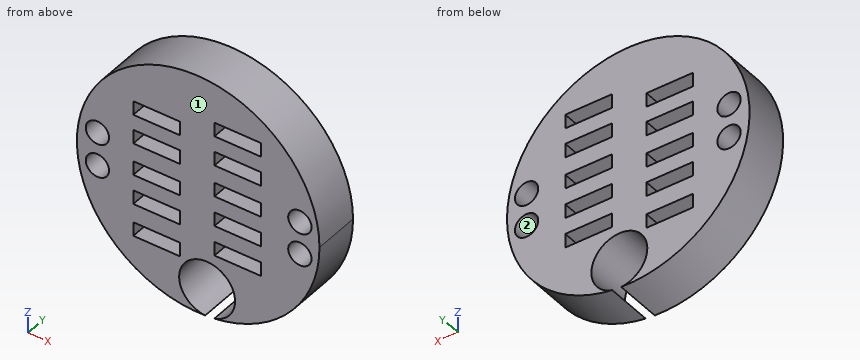
Autodesk Inventor part; units mm, degrees
ref_plane "YZ Plane" through (0, 0, 0) normal (1, 0, 0) x (0, 1, 0)
ref_plane "XZ Plane" through (0, 0, 0) normal (0, 1, 0) x (-1, 0, 0)
ref_plane "XY Plane" through (0, 0, 0) normal (0, 0, 1) x (1, 0, 0)
sketch "Sketch3" plane through (0, 0, 0) normal (0, 1, 0) x (-1, 0, 0)
  circle A0 centre (0, 0) radius 13.5
  line L0 (-6.7499, 8.6501) -> (-1.7499, 8.6501)
  line L1 (-1.7499, 8.6501) -> (-1.7499, 7.1501)
  line L2 (-1.7499, 7.1501) -> (-6.7499, 7.1501)
  line L3 (-6.7499, 7.1501) -> (-6.7499, 8.6501)
  line L4 (-6.75, 5.45) -> (-1.7499, 5.45)
  line L5 (-1.7499, 5.45) -> (-1.7499, 3.95)
  line L6 (-1.7499, 3.95) -> (-6.75, 3.95)
  line L7 (-6.75, 3.95) -> (-6.75, 5.45)
  line L8 (-6.75, 2.0498) -> (-1.75, 2.0498)
  line L9 (-1.75, 2.0498) -> (-1.75, 0.5498)
  line L10 (-1.75, 0.5498) -> (-6.75, 0.5498)
  line L11 (-6.75, 0.5498) -> (-6.75, 2.0498)
  line L12 (-6.75, -1.2) -> (-1.75, -1.2)
  line L13 (-1.75, -1.2) -> (-1.75, -2.7)
  line L14 (-1.75, -2.7) -> (-6.75, -2.7)
  line L15 (-6.75, -2.7) -> (-6.75, -1.2)
  line L16 (-6.75, -4.4501) -> (-1.75, -4.4501)
  line L17 (-1.75, -4.4501) -> (-1.75, -5.9501)
  line L18 (-1.75, -5.9501) -> (-6.75, -5.9501)
  line L19 (-6.75, -5.9501) -> (-6.75, -4.4501)
  line L20 (1.9499, 7.1) -> (6.9499, 7.1)
  line L21 (6.9499, 7.1) -> (6.9499, 5.6)
  line L22 (6.9499, 5.6) -> (1.9499, 5.6)
  line L23 (1.9499, 5.6) -> (1.9499, 7.1)
  line L24 (1.9499, 3.95) -> (6.9499, 3.95)
  line L25 (6.9499, 3.95) -> (6.9499, 2.45)
  line L26 (6.9499, 2.45) -> (1.9499, 2.45)
  line L27 (1.9499, 2.45) -> (1.9499, 3.95)
  line L28 (1.9499, 0.5004) -> (6.9499, 0.5004)
  line L29 (6.9499, 0.5004) -> (6.9499, -0.9996)
  line L30 (6.9499, -0.9996) -> (1.9499, -0.9996)
  line L31 (1.9499, -0.9996) -> (1.9499, 0.5004)
  line L32 (1.9499, -2.7) -> (6.9499, -2.7)
  line L33 (6.9499, -2.7) -> (6.9499, -4.2)
  line L34 (6.9499, -4.2) -> (1.9499, -4.2)
  line L35 (1.9499, -4.2) -> (1.9499, -2.7)
  line L36 (1.9499, -6.1999) -> (6.9499, -6.1999)
  line L37 (6.9499, -6.1999) -> (6.9499, -7.6999)
  line L38 (6.9499, -7.6999) -> (1.9499, -7.6999)
  line L39 (1.9499, -7.6999) -> (1.9499, -6.1999)
  point P0 (-6.7499, 7.9001)
  point P1 (-6.75, 4.7)
  point P2 (-5.95, -5.2001)
  dimension "d3" = 27
  dimension "d4" = 5
  dimension "d5" = 1.5
  dimension "d6" = 1.5
  dimension "d7" = 5
  dimension "d8" = 1.5
  dimension "d9" = 5
  dimension "d10" = 1.5
  dimension "d11" = 5
  dimension "d12" = 1.5
  dimension "d13" = 0.8
  dimension "d14" = 5
  dimension "d15" = 1.5
  dimension "d16" = 5
  dimension "d17" = 1.5
  dimension "d18" = 5
  dimension "d19" = 1.5
  dimension "d20" = 5
  dimension "d21" = 1.5
  dimension "d22" = 1.5
extrude "Extrusion1" add sketch "Sketch3" along normal blind 5
sketch "Sketch4" plane through (0, 5, 0) normal (0, 1, 0) x (1, 0, 0)
  circle A0 centre (-10.8, -1.9) radius 0.75
  circle A1 centre (-10.8, 1.7) radius 0.75
  circle A2 centre (10.9, -1.85) radius 0.75
  circle A3 centre (10.9, 1.65) radius 0.75
  circle A4 centre (0.958, 9.985) radius 3
  point P0 (0, 0)
  dimension "d25" = 1.5
  dimension "d26" = 1.5
  dimension "d27" = 1.5
  dimension "d28" = 1.5
  dimension "d29" = 6
extrude "Extrusion2" cut sketch "Sketch4" against normal blind 5
sketch "Sketch5" plane through (0, 5, 0) normal (0, 1, 0) x (1, 0, 0)
  circle A0 centre (-10.8, -1.9) radius 0.75
  circle A1 centre (-10.8, -1.9) radius 1.25
  circle A2 centre (-10.8, 1.7) radius 0.75
  circle A3 centre (-10.8, 1.7) radius 1.25
  circle A4 centre (10.9, -1.85) radius 0.75
  circle A5 centre (10.9, -1.85) radius 1.25
  circle A6 centre (10.9, 1.65) radius 0.75
  circle A7 centre (10.9, 1.65) radius 1.25
  point P0 (0, 0)
  dimension "d33" = 2.5
  dimension "d34" = 2.5
  dimension "d35" = 2.5
  dimension "d36" = 2.5
extrude "Extrusion3" cut sketch "Sketch5" against normal blind 5 contours A0 | A1 | A2 | A3 | A4 | A5 | A6 | A7
sketch "Sketch6" plane through (0, 5, 0) normal (0, 1, 0) x (1, 0, 0)
  circle A0 centre (0, 0) radius 13.5
  circle A1 centre (0, 0) radius 13
  dimension "d41" = 26
extrude "Extrusion4" cut sketch "Sketch6" against normal blind 10
properties part number "Seperator_V2_3DPrint"
Can you work these out from the model? Positions are in its coordinate system, mm. Face numbers are marked on the shaded views. Coordinates: 2 decimals unless noted, no trailing zeros. Order: outer loops, then holes, each group sorted by start corner. A loop starts at its lowest first (then second) coordinate and runs counter-clockwise, first axis right, second up. Notation, with made-up numbers: (38.5, 28) - (90.5, 28) arc R15 cw to (90.5, 37) - close; hole circle Ø10 at (65.5, -22.75). An arc over 180 degrees is marked (long way). Answer as a JSON object with one key per item and string values. Group by question number.
Q1. Imagine slicing it at B-B (z = 2.75). Please give me the cut outline in (x, y).
Q2. Imagine slicing it at D-D (x = 0). Please give me the cut outline in (y, z).
Q3. Imagine slicing it at A-A (x = -10.8). Please give me the cut outline in (y, z), and give its area (3 significant figures).
Q4. Will these pins go through, and if not, where does the flat tip stop? P1, Ø0.8, axis at y = 3.5, z = 8, coming from the -X side; P2, Ø3, axis at y = 4, z = 5.5, coming from the +X side; P3, Ø2, axis at y = 2, z = -2, coming from the -X side.
Q5. We'd pull the mould along Z, two halves only. Please class the marked faces 1 and 2: +Z half, -Z half, draft (parallel to the pull), parting line (faces both ways), or undercut.
Q6. I need wall thicknesses on line 1 (X direction, y = 1.25, z = 0); line 2 (Z direction, x = 11.75, y = 0.7); line 3 (X direction, y = 4.7, z = 1.25). Which ranges of each line are inside material? Lowest first, please. Write a range as from..to.
Q7. Imagine slicing it at C-C (x = -5.5). Please give me the cut outline in (y, z), and give its area (3 significant figures).
Determined:
{
 "1": {"outline": "(-12.71, 0) - (-11.72, 0) - (-11.72, 5) - (-12.71, 5) - close; (-9.88, 0) - (-6.95, 0) - (-6.95, 5) - (-9.88, 5) - close; (-1.95, 0) - (10.03, 0) - (10.03, 5) - (-1.95, 5) - close; (11.77, 0) - (12.71, 0) - (12.71, 5) - (11.77, 5) - close"},
 "2": {"outline": "(0, -13) - (5, -13) - (5, -12.83) - (0, -12.83) - close; (0, -7.14) - (5, -7.14) - (5, 13) - (0, 13) - close"},
 "3": {"outline": "(0, -7.24) - (5, -7.24) - (5, -2.95) - (0, -2.95) - close; (0, -0.45) - (5, -0.45) - (5, 0.65) - (0, 0.65) - close; (0, 3.15) - (5, 3.15) - (5, 7.24) - (0, 7.24) - close", "area": "47.4 mm2"},
 "4": {"P1": "stops at x = -10.55", "P2": "stops at x = 12.37", "P3": "stops at x = -12.96"},
 "5": {"face 1": "draft", "face 2": "undercut"},
 "6": {"line 1": "x = -13..-6.95, -1.95..13", "line 2": "z = -5.56..-2.57, -0.73..0.93, 2.77..5.56", "line 3": "x = -12.94..-11.87, -9.73..1.75, 6.75..9.8, 12..12.94"},
 "7": {"outline": "(0, -11.78) - (5, -11.78) - (5, -7.7) - (0, -7.7) - close; (0, -6.2) - (5, -6.2) - (5, -4.2) - (0, -4.2) - close; (0, -2.7) - (5, -2.7) - (5, -1) - (0, -1) - close; (0, 0.5) - (5, 0.5) - (5, 2.45) - (0, 2.45) - close; (0, 3.95) - (5, 3.95) - (5, 5.6) - (0, 5.6) - close; (0, 7.1) - (5, 7.1) - (5, 11.78) - (0, 11.78) - close", "area": "80.3 mm2"}
}
